from build123d import *

# Parameters (mm, degrees)
SKETCH1_R           = 9
BOSS_EXTRUDE1_DEPTH = 3.175
BOSS_EXTRUDE2_DEPTH = 11
SKETCH3_R           = 6.399999954
BOSS_EXTRUDE3_DEPTH = 2
SKETCH4_R           = 3.899999974
BOSS_EXTRUDE4_DEPTH = 6.999999906
BOSS_EXTRUDE5_DEPTH = 3.175
BOSS_EXTRUDE7_DEPTH = 4
SKETCH8_R           = 2
CUT_EXTRUDE1_DEPTH  = 4
SKETCH9_R           = 1.650000048
CUT_EXTRUDE2_DEPTH  = 12.175
SKETCH10_R          = 4
CUT_EXTRUDE3_DEPTH  = 2.2
SKETCH11_R          = 1.7145
CUT_EXTRUDE4_DEPTH  = 1.5


with BuildPart() as part:
    # Sketch1 → Boss-Extrude1 (new body)
    with BuildSketch(Plane(origin=(0, 0, 0), x_dir=(1, 0, 0), z_dir=(0, 1, 0))):
        Circle(SKETCH1_R)
    extrude(amount=BOSS_EXTRUDE1_DEPTH)

    # Sketch2 → Boss-Extrude2 (add)
    with BuildSketch(Plane(origin=(0, 3.175, 0), x_dir=(1, 0, 0), z_dir=(0, 1, 0))):
        with BuildLine():
            Line((-7.707704384, -4.646643211), (-5.138469589, -3.097762141))
            ThreePointArc((-5.138469589, -3.097762141), (0, 6), (5.138469589, -3.097762141))
            Line((5.138469589, -3.097762141), (7.707704384, -4.646643211))
            ThreePointArc((7.707704384, -4.646643211), (0, 9), (-7.707704384, -4.646643211))
        make_face()
    extrude(amount=BOSS_EXTRUDE2_DEPTH)

    # Sketch3 → Boss-Extrude3 (add)
    with BuildSketch(Plane.XZ):
        Circle(SKETCH3_R)
    extrude(amount=BOSS_EXTRUDE3_DEPTH)

    # Sketch4 → Boss-Extrude4 (add)
    with BuildSketch(Plane.XZ.offset(2)):
        Circle(SKETCH4_R)
    extrude(amount=BOSS_EXTRUDE4_DEPTH)

    # Sketch6 → Boss-Extrude5 (add)
    with BuildSketch(Plane(origin=(0, 0, 0), x_dir=(1, 0, 0), z_dir=(0, 1, 0))):
        with BuildLine():
            Line((-9, 0), (-9, 13.194197425))
            ThreePointArc((-9, 13.194197425), (-4.5, 17.694197425), (0, 13.194197425))
            Line((0, 13.194197425), (0, 9))
            ThreePointArc((0, 9), (-6.363961031, 6.363961031), (-9, 0))
        make_face()
    extrude(amount=BOSS_EXTRUDE5_DEPTH)

    # Sketch7 → Boss-Extrude7 (add)
    with BuildSketch(Plane(origin=(0, 8.174999906, 0), x_dir=(1, 0, 0), z_dir=(0, 1, 0))):
        with BuildLine():
            Line((0, 9), (0, 13.194197425))
            ThreePointArc((0, 13.194197425), (-4.5, 17.694197425), (-9, 13.194197425))
            Line((-9, 13.194197425), (-9, 0))
            ThreePointArc((-9, 0), (-6.363961031, 6.363961031), (0, 9))
        make_face()
    extrude(amount=BOSS_EXTRUDE7_DEPTH)

    # Sketch8 → Cut-Extrude1 (cut)
    with BuildSketch(Plane(origin=(0, 12.174999906, 0), x_dir=(1, 0, 0), z_dir=(0, 1, 0))):
        with Locations((-4.5, 13.194197425)):
            Circle(SKETCH8_R)
    extrude(amount=-CUT_EXTRUDE1_DEPTH, mode=Mode.SUBTRACT)

    # Sketch9 → Cut-Extrude2 (cut)
    with BuildSketch(Plane(origin=(0, 3.175, 0), x_dir=(1, 0, 0), z_dir=(0, 1, 0))):
        Circle(SKETCH9_R)
    extrude(amount=-CUT_EXTRUDE2_DEPTH, mode=Mode.SUBTRACT)

    # Sketch10 → Cut-Extrude3 (cut)
    with BuildSketch(Plane(origin=(0, 3.175, 0), x_dir=(1, 0, 0), z_dir=(0, 1, 0))):
        Circle(SKETCH10_R)
    extrude(amount=-CUT_EXTRUDE3_DEPTH, mode=Mode.SUBTRACT)

    # Sketch11 → Cut-Extrude4 (cut)
    with BuildSketch(Plane(origin=(0, 3.175, 0), x_dir=(1, 0, 0), z_dir=(0, 1, 0))):
        with Locations((-4.5, 13.194197425)):
            Circle(SKETCH11_R)
    extrude(amount=-CUT_EXTRUDE4_DEPTH, mode=Mode.SUBTRACT)


solid = part.part
Here's how the part is built. I have some questions about the finished solid (model axes, mm). A direction names the side the tool comes from. Round coordinates to 2 decimals unless told otherwise and drop trailing zeros. Loops run counter-clockwise (first coordinate to the right, second up) from the corner with the lowest first, then second, coordinate; pieces in that order, holes last.
1. Which directions (+Z, -Z, +X, -X, +Y, -Y) give clear straight access to the entire face, cutting with the end or side of a thin tool? Please do faces 1 (the face through (-5, 1.675, -13)), 2 (the face through (-4, 3.175, -11)), 3 (the face through (6.405, 8.598, 3.861)).
Answer list:
face 1: +Y
face 2: -Z, -X
face 3: +Z, +Y
2. If we section it at B-B on x = -4.5: Write out the boundary of the cut face in (y, z) (3 decimals), plus the area to 3 significant figures.
Answer list:
outline: (-2, -4.551) - (0, -4.551) - (0, -17.694) - (3.175, -17.694) - (3.175, -14.909) - (1.675, -14.909) - (1.675, -11.48) - (3.175, -11.48) - (3.175, -7.794) - (8.175, -7.794) - (8.175, -11.194) - (12.175, -11.194) - (12.175, -7.794) - (14.175, -7.794) - (14.175, -3.969) - (3.175, -3.969) - (3.175, 7.794) - (0, 7.794) - (0, 4.551) - (-2, 4.551) - close; (8.175, -17.694) - (12.175, -17.694) - (12.175, -15.194) - (8.175, -15.194) - close
area: 160 mm2
3. If we section it at C-C on y = 2.25: Write out the boundary of the cut face in (x, z), plus the area to 3 significant figures.
Answer list:
outline: (-9, -13.19) arc R4.5 ccw to (0, -13.19) - (0, -9) arc R9 ccw (long way) to (-9, 0) - close; hole circle Ø3.43 at (-4.5, -13.19); hole circle Ø8 at (0, 0)
area: 282 mm2
4. If we section it at A-A on y = 8.5: Write out the boundary of the cut face in (x, z).
Answer list:
outline: (-9, -13.19) arc R4.5 ccw to (0, -13.19) - (0, -9) arc R9 ccw to (7.71, 4.65) - (5.14, 3.1) arc R6 cw (long way) to (-5.14, 3.1) - (-7.71, 4.65) arc R9 ccw to (-9, 0) - close; hole circle Ø4 at (-4.5, -13.19)
5. We'd pull the mould along Z, two halves only. Please class faces 4 (the face through (-9, 2, -7)), 5 (the face through (-4.93, 10.2, -11.24)), 6 (the face through (-1.387, -0.986, -6.248)): +Z half, -Z half, draft (parallel to the pull), parting line (faces both ways), or undercut.
Answer list:
face 4: draft
face 5: undercut
face 6: parting line
6. If I drill on line 1 along X through (y, z) = (12.75, 0.25); line 2 along Y through (x, z) = (-6.5, -9.25) (3 decimals); line 3 along Y through (x, z) = (-3, -13.25) (3 decimals), over which ranges is the centre line in solid material (lowest first)?
Answer list:
line 1: x = -9 to -5.99, 5.99 to 9
line 2: y = 0 to 3.175, 8.175 to 12.175
line 3: y = 0 to 1.675
7. For P1, Ø4.5, axis at x = -2.5, z = -10, coming from the -Y side; P2, Ø2.5, axis at x = -4, z = -13, coming from the +Y side (3 decimals); P3, Ø2, axis at x = -4.5, z = -13.19, coming from the +Y side (3 decimals), each with a flat end and sliding along its axis, tell me the tip position at first contact or that it passes through.
Answer list:
P1: stops at y = 0
P2: stops at y = 3.175
P3: stops at y = 1.675
8. If we section it at D-D on z = 5.5: Write out the boundary of the cut face in (x, y) (3 decimals).
Answer list:
outline: (-7.124, 0) - (-3.273, 0) - (-3.273, -2) - (3.273, -2) - (3.273, 0) - (7.124, 0) - (7.124, 3.175) - (-7.124, 3.175) - close
